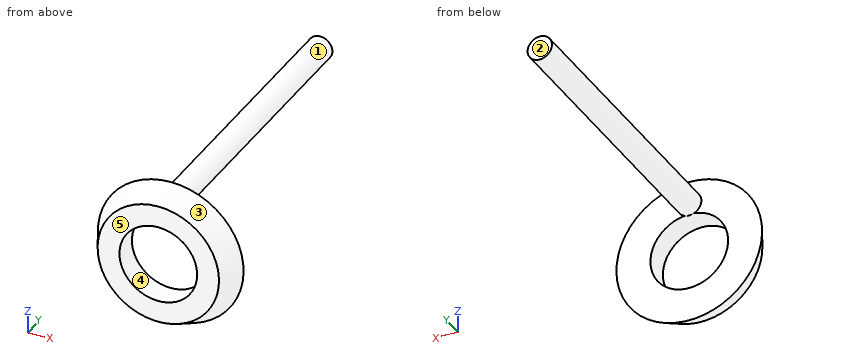
```python
from build123d import *

# Parameters (mm, degrees)
SKETCH1_R           = 3
BOSS_EXTRUDE1_DEPTH = 1
SKETCH2_R           = 1.6
CUT_EXTRUDE1_DEPTH  = 1
SKETCH3_R           = 0.5
BOSS_EXTRUDE2_DEPTH = 12
CHAMFER1_SIZE       = 1
CHAMFER1_SIZE_2     = 0.5


with BuildPart() as part:
    # Sketch1 → Boss-Extrude1 (new body)
    with BuildSketch(Plane(origin=(0, 0, 0), x_dir=(1, 0, 0), z_dir=(0, 1, 0))):
        with Locations(Location((0, 0, 0), (0, 0, 270))):
            Circle(SKETCH1_R)
    extrude(amount=BOSS_EXTRUDE1_DEPTH)

    # Sketch2 → Cut-Extrude1 (cut)
    with BuildSketch(Plane(origin=(0, 1, 0), x_dir=(1, 0, 0), z_dir=(0, 1, 0))):
        with Locations(Location((0, 0, 0), (0, 0, 270))):
            Circle(SKETCH2_R)
    extrude(amount=-CUT_EXTRUDE1_DEPTH, mode=Mode.SUBTRACT)

    # Sketch3 → Boss-Extrude2 (add)
    with BuildSketch(Plane(origin=(0, 1, 0), x_dir=(1, 0, 0), z_dir=(0, 1, 0))):
        with Locations(Location((0, -2.048388822, 0), (0, 0, 112.975296156))):
            Circle(SKETCH3_R)
    extrude(amount=BOSS_EXTRUDE2_DEPTH)

    # Chamfer1
    # the kernel refuses this chamfer: 1, 0.5 mm, written as the material it takes off along each edge
    with BuildSketch(Plane(origin=(0, 0, 0), x_dir=(0, 0, 1), z_dir=(-1, 0, 0))) as chamfer1_piece_1:
        Polygon((3, CHAMFER1_SIZE), (3 - CHAMFER1_SIZE_2, 0), (3, 0), align=None)
    revolve(axis=Axis((0, 0, 0), (0, 1, 0)), mode=Mode.SUBTRACT)


solid = part.part
```
Verification items for the finished model (mm, model axes). Face numbers are marked on the shaded views. A direction names the side the tool comes from. Give positions to 0.01 mm unless a question says otherwise; leave off trailing zeros. Order: outer loops, then holes, each group sorted by start corner. A loop starts at its lowest first (then second) coordinate and runs counter-clockwise, first axis right, second up. Notation, with made-up numbers: (16.25, 88.5) -> (36.25, 88.5) arc R31 ccw to (36.25, 116.5) -> close; hole circle Ø6 at (61.5, 42.5). An arc over 180 degrees is marked (long way). Use a Markdown table: item, result.
1) Tool access check on the marked faces 1 and 2. Record the directions out of +Z, -Z, +X, -X, +Y, -Y that give a thin tool (end or side, any length) a straight path to the whole face; none if there is none.
Results:
| item | result |
|---|---|
| face 1 | +Y |
| face 2 | +Z, -Z, +X, -X, +Y |
2) Section check B-B, the plane x = 0. Record the boundary of the cut face in (y, z), then the cut area to 3 significant figures.
Results:
| item | result |
|---|---|
| outline | (0, -2.5) -> (1, -3) -> (1, -1.6) -> (0, -1.6) -> close; (0, 1.6) -> (1, 1.6) -> (1, 1.55) -> (13, 1.55) -> (13, 2.55) -> (1, 2.55) -> (1, 3) -> (0, 2.5) -> close |
| area | 14.3 mm² |
3) Mould release check, pull along Z, two halves, no side actions. Record for the marked faces 3, 4 and 5: pulls with the +Z half, pulls with the -Z half, needs draft (parallel to the pull), parting line crosses it, or undercut.
Results:
| item | result |
|---|---|
| face 3 | parting line crosses it |
| face 4 | undercut |
| face 5 | needs draft |
4) Material ranges on probe 1 along Y at (x, z) = (-0.9, -1.95); probe 2 along Z at (x, y) = (0, 0.4); probe 3 along Z at (x, y) = (0, 0.6), recorded low to high.
Results:
| item | result |
|---|---|
| probe 1 | 0 to 1 |
| probe 2 | -2.7 to -1.6, 1.6 to 2.7 |
| probe 3 | -2.8 to -1.6, 1.6 to 2.8 |
5) Section check A-A, the plane z = 0. Record the boundary of the cut face in (x, y).
Results:
| item | result |
|---|---|
| outline | (-3, 1) -> (-2.5, 0) -> (-1.6, 0) -> (-1.6, 1) -> close; (1.6, 0) -> (2.5, 0) -> (3, 1) -> (1.6, 1) -> close |
6) Section check C-C, the plane y = 8. Record the boundary of the cut face in (x, z), then the cut area to 3 significant figures.
Results:
| item | result |
|---|---|
| outline | circle Ø1 at (0, 2.05) |
| area | 0.785 mm² |
7) Depth check by flat-ended pin: pin 1 Ø1.5 at (x, z) = (-2.5, 2) entering from +Y; pin 2 Ø1.5 at (y, z) = (10.5, -1) entering from +X. Enter the tip coordinate at first touch or a pass-through.
Results:
| item | result |
|---|---|
| pin 1 | y = 1 |
| pin 2 | through |
